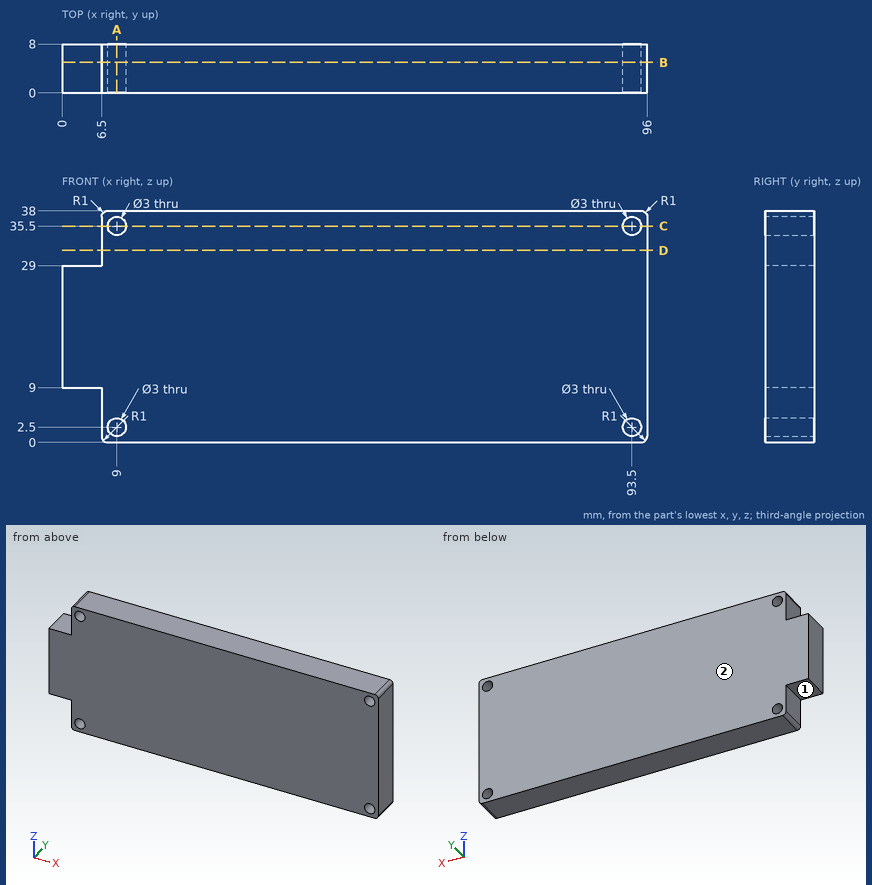
Could you check a few things on this drawing? It's one solid part, dimensions in mm from its lowest x, y, z. A direction names the side the tool comes from. Coordinates: 2 decimals unless noted, no trailing zeros. Order: outer loops, then holes, each group sorted by start corner. A loop starts at its lowest first (then second) coordinate and runs counter-clockwise, first axis right, second up. Notation, with made-up numbers: (74.25, 47.5) -> (96.25, 47.5) arc R21 ccw to (96.25, 54.5) -> close; hole circle Ø6 at (87.5, 40.25). An arc over 180 degrees is marked (long way). Answer in a Markdown table with one row per item.
(1) I want a section at A-A on x = 9. List the corners of the cut face in (y, z) for me, then the cut area to 3 significant figures.
Answer key:
| item | result |
|---|---|
| outline | (0, 0) -> (8, 0) -> (8, 1) -> (0, 1) -> close; (0, 4) -> (8, 4) -> (8, 34) -> (0, 34) -> close; (0, 37) -> (8, 37) -> (8, 38) -> (0, 38) -> close |
| area | 256 mm^2 |
(2) I want a section at C-C on z = 35.5. List the corners of the cut face in (x, y) for me, then the cut area to 3 significant figures.
Answer key:
| item | result |
|---|---|
| outline | (6.5, 0) -> (7.5, 0) -> (7.5, 8) -> (6.5, 8) -> close; (10.5, 0) -> (92, 0) -> (92, 8) -> (10.5, 8) -> close; (95, 0) -> (96, 0) -> (96, 8) -> (95, 8) -> close |
| area | 668 mm^2 |
(3) I want a section at B-B on y = 5. List the corners of the cut face in (x, z) for me.
Answer key:
| item | result |
|---|---|
| outline | (0, 9) -> (6.5, 9) -> (6.5, 1) arc R1 ccw to (7.5, 0) -> (95, 0) arc R1 ccw to (96, 1) -> (96, 37) arc R1 ccw to (95, 38) -> (7.5, 38) arc R1 ccw to (6.5, 37) -> (6.5, 29) -> (0, 29) -> close; hole circle Ø3 at (9, 2.5); hole circle Ø3 at (9, 35.5); hole circle Ø3 at (93.5, 2.5); hole circle Ø3 at (93.5, 35.5) |
(4) Please list where these lines run through material, in increasing order: probe 1 along X at (y, z) = (3.75, 35.5); probe 2 along X at (y, z) = (2.5, 6); probe 3 along Z at (x, y) = (7, 3.25).
Answer key:
| item | result |
|---|---|
| probe 1 | 6.5 to 7.5, 10.5 to 92, 95 to 96 |
| probe 2 | 6.5 to 96 |
| probe 3 | 0.13 to 37.87 |
(5) On a 3-axis mill with a long thin cutter (end or side, diameter ignored), from which of +Z, -Z, +X, -X, +Y, -Y can I reach the whole of each face in a straight line? I mean the marked faces 1 and 2. Say none if no direction works.
Answer key:
| item | result |
|---|---|
| face 1 | -Z, -X, +Y, -Y |
| face 2 | +Z, -Z, +X, -X, +Y |
(6) Will these pins go through, and if not, where does the flat tip stop? pin 1 Ø2.5 at (x, z) = (93.5, 35.5) entering from -Y; pin 2 Ø3 at (x, y) = (4.5, 2) entering from -Z; pin 3 Ø4 at (y, z) = (4.5, 4.5) entering from -X.
Answer key:
| item | result |
|---|---|
| pin 1 | through |
| pin 2 | z = 9 |
| pin 3 | x = 6.5 |
(7) I want a section at D-D on z = 31.5. List the corners of the cut face in (x, y) for me, then the cut area to 3 significant figures.
Answer key:
| item | result |
|---|---|
| outline | (6.5, 0) -> (96, 0) -> (96, 8) -> (6.5, 8) -> close |
| area | 716 mm^2 |
